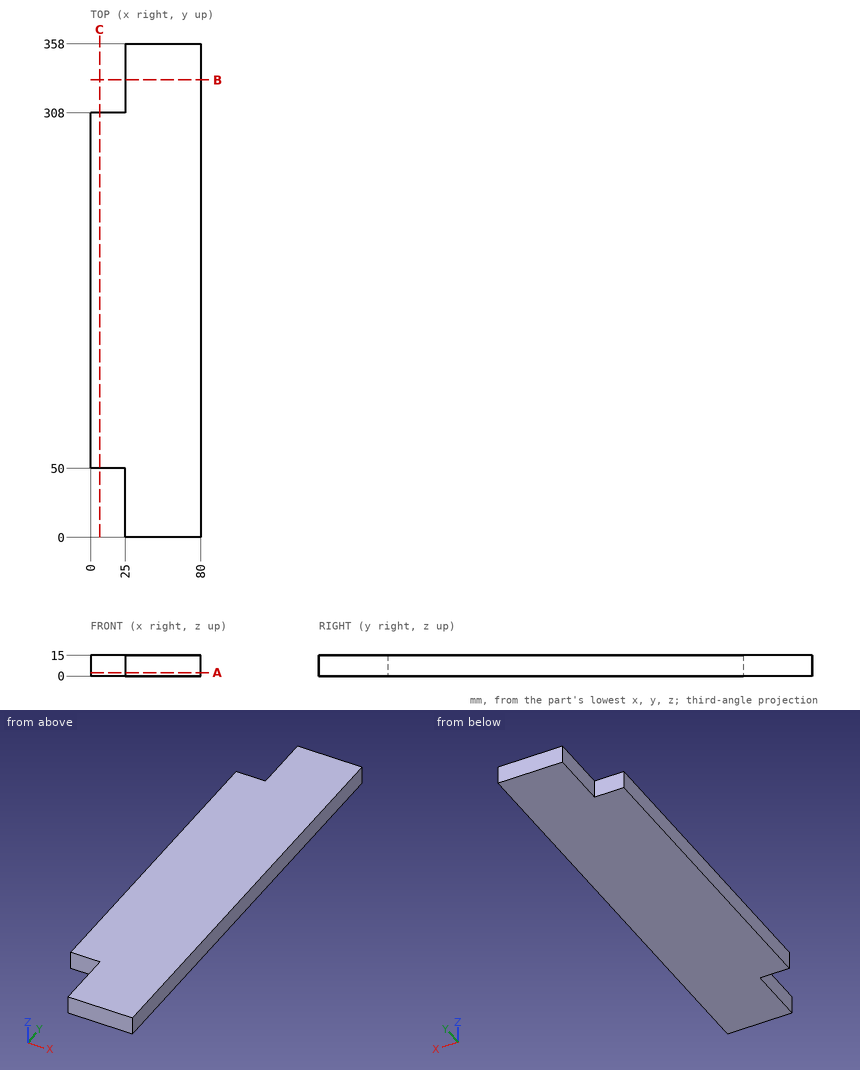
Here's the drawing with two shaded views (mm, measured from the low corner). I have some questions. Give positions to 0.01 mm unless a question says otherwise; leave off trailing zeros. Write each loop counter-clockwise with the first axis right and the second up, starting at its lowest first coordinate (ties: lowest second). Pieces come first, ordered by that corner, then holes. Notation, with made-up numbers: (-28.5, 53.25) -> (6.5, 53.25) arc R19 cw to (6.5, 70.25) -> close; hole circle Ø3 at (-8, 44). An arc over 180 degrees is marked (long way). Use one line per item in the form item = value.
1) Suppose I cut it at B-B (y = 332). Please give me the cut outline in (x, z), and give its area (3 significant figures).
Verdict:
outline = (25, 0) -> (80, 0) -> (80, 15) -> (25, 15) -> close
area = 825 mm2
2) If I drill on L1, parallel to X at y = 48, z = 13; L2, parallel to Y at x = 6.5, z = 4, over which ranges is the centre line in solid material (lowest first)? Write a range as [from, to].
Verdict:
L1 = [25, 80]
L2 = [50, 308]
3) I'm going to push flat-ended pins straight in: pin 1 (4 mm diameter, centred on x = 21.5, z = 2.5, fed in from -Y); pin 2 (4.5 mm diameter, centred on x = 18, z = 9, fed in from +Y). Where does each tip first touch, or does it pass through?
Verdict:
pin_1 = 50
pin_2 = 308
4) Suppose I cut it at C-C (x = 6.5). Please give me the cut outline in (y, z), and give its area (3 significant figures).
Verdict:
outline = (50, 0) -> (308, 0) -> (308, 15) -> (50, 15) -> close
area = 3,870 mm2
5) Suppose I cut it at A-A (z = 2.5). Please give me the cut outline in (x, y), and give its area (3 significant figures).
Verdict:
outline = (0, 50) -> (25, 50) -> (25, 0) -> (80, 0) -> (80, 358) -> (25, 358) -> (25, 308) -> (0, 308) -> close
area = 26,100 mm2
